from build123d import *

# Parameters (mm, degrees)
SKETCH_R      = 9
SKETCH_R_2    = 2.55
PAD_DEPTH     = 1.6
SKETCH001_R   = 3.15
SKETCH001_R_2 = 2.55
PAD001_DEPTH  = 5.85


with BuildPart() as part:
    # Sketch → Pad (new body)
    with BuildSketch(Plane.XY):
        Circle(SKETCH_R)
        Circle(SKETCH_R_2, mode=Mode.SUBTRACT)
    extrude(amount=-PAD_DEPTH)

    # Sketch001 → Pad001 (new body)
    with BuildSketch(Plane(origin=(0, 0, -1.6), x_dir=(1, 0, 0), z_dir=(0, 0, -1))):
        Circle(SKETCH001_R)
        Circle(SKETCH001_R_2, mode=Mode.SUBTRACT)
    extrude(amount=PAD001_DEPTH)


solid = part.part
Geometry check sheet. Reference: the model listing, model coordinates, mm. A direction names the side the tool comes from. Round coordinates to 2 decimals unless told otherwise and drop trailing zeros. Loops run counter-clockwise (first coordinate to the right, second up) from the corner with the lowest first, then second, coordinate; pieces in that order, holes last.
Item 1: Gauge pin test, flat ends, axial feed: pin 1 (8 mm diameter, centred on x = -6, y = 6, fed in from -Z); pin 2 (3 mm diameter, centred on x = 3, z = -6.5, fed in from +Y). Record the tip position at first contact, or that the pin passes through.
Item 2: Cross-section at A-A on x = 0. Record the boundary of the cut face in (y, z).
Item 3: Cross-section at D-D on y = 4. Record the boundary of the cut face in (x, z).
Item 4: Cross-section at B-B on z = -1. Record the boundary of the cut face in (x, y).
Item 5: Access from +Z, -Z, +X, -X, +Y, -Y to the whole of each face (thin tool, end or side, straight path). Record for faces 1 (the flat face through (0, -4, -1.6)), 2 (the flat face through (2, -2, 0)).
Item 6: Cross-section at C-C on z = -3.25. Record the boundary of the cut face in (x, y), then the cut area to 3 significant figures.
Item 7: Thickness scan on line 1 (Y direction, x = 0, z = -6.15); line 2 (Y direction, x = 0, z = -0.8). Record the ranges inside material, lowest first.
Answer sheet:
1. pin 1: stops at z = -1.6
1. pin 2: stops at y = 2.77
2. outline: (-9, -1.6) - (-3.15, -1.6) - (-3.15, -7.45) - (-2.55, -7.45) - (-2.55, 0) - (-9, 0) - close; (2.55, -7.45) - (3.15, -7.45) - (3.15, -1.6) - (9, -1.6) - (9, 0) - (2.55, 0) - close
3. outline: (-8.06, -1.6) - (8.06, -1.6) - (8.06, 0) - (-8.06, 0) - close
4. outline: circle Ø18 at (0, 0); hole circle Ø5.1 at (0, 0)
5. face 1: -Z
5. face 2: +Z, +X, -X, +Y, -Y
6. outline: circle Ø6.3 at (0, 0); hole circle Ø5.1 at (0, 0)
6. area: 10.7 mm2
7. line 1: y = -3.15 to -2.55, 2.55 to 3.15
7. line 2: y = -9 to -2.55, 2.55 to 9
